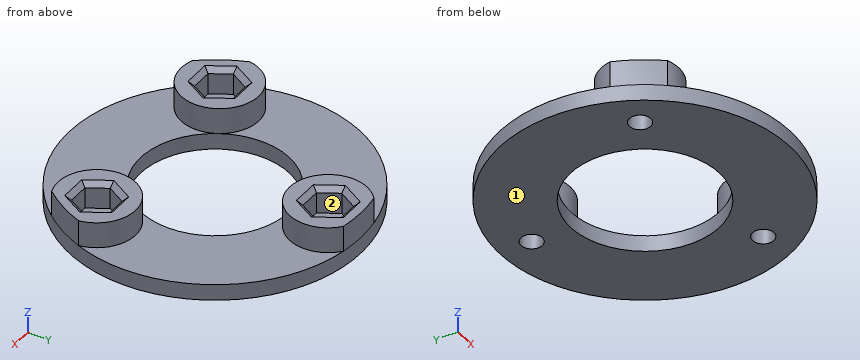
from build123d import *

# Parameters (mm, degrees)
SKETCH1_R           = 22.5
SKETCH1_R_2         = 11.5
SKETCH1_R_3         = 1.65
BOSS_EXTRUDE1_DEPTH = 2.5
BOSS_EXTRUDE2_DEPTH = 4
CHAMFER1_SIZE       = 0.75


with BuildPart() as part:
    # Sketch1 → Boss-Extrude1 (new body)
    with BuildSketch(Plane.XY):
        Circle(SKETCH1_R)
        Circle(SKETCH1_R_2, mode=Mode.SUBTRACT)
        with Locations((0, 17.5)):
            Circle(SKETCH1_R_3, mode=Mode.SUBTRACT)
        with Locations((15.155444566, -8.75)):
            Circle(SKETCH1_R_3, mode=Mode.SUBTRACT)
        with Locations((-15.155444566, -8.75)):
            Circle(SKETCH1_R_3, mode=Mode.SUBTRACT)
    extrude(amount=BOSS_EXTRUDE1_DEPTH)

    # Sketch2 → Boss-Extrude2 (add)
    # profile 1 of 3: a face of its own
    with BuildSketch(Plane.XY.offset(2.5)):
        with BuildLine():
            ThreePointArc((3.747543413, 22.185714286), (0, 22.5), (-3.747543413, 22.185714286))
            ThreePointArc((-3.747543413, 22.185714286), (0, 11.5), (3.747543413, 22.185714286))
        make_face()
        Polygon((1.659882024, 20.375), (3.319764048, 17.5), (1.659882024, 14.625), (-1.659882024, 14.625), (-3.319764048, 17.5), (-1.659882024, 20.375), align=None, mode=Mode.SUBTRACT)
    # profile 2 of 3: a face of its own
    with BuildSketch(Plane.XY.offset(2.5)):
        with BuildLine():
            ThreePointArc((-17.339620466, -14.33832494), (-9.959292144, -5.75), (-21.087163879, -7.847389345))
            ThreePointArc((-21.087163879, -7.847389345), (-19.485571585, -11.25), (-17.339620466, -14.33832494))
        make_face()
        Polygon((-18.475208614, -8.75), (-16.81532659, -5.875), (-13.495562542, -5.875), (-11.835680518, -8.75), (-13.495562542, -11.625), (-16.81532659, -11.625), align=None, mode=Mode.SUBTRACT)
    # profile 3 of 3: a face of its own
    with BuildSketch(Plane.XY.offset(2.5)):
        with BuildLine():
            ThreePointArc((17.339620466, -14.33832494), (19.485571585, -11.25), (21.087163879, -7.847389345))
            ThreePointArc((21.087163879, -7.847389345), (9.959292144, -5.75), (17.339620466, -14.33832494))
        make_face()
        Polygon((16.81532659, -11.625), (13.495562542, -11.625), (11.835680518, -8.75), (13.495562542, -5.875), (16.81532659, -5.875), (18.475208614, -8.75), align=None, mode=Mode.SUBTRACT)
    extrude(amount=BOSS_EXTRUDE2_DEPTH)

    # Chamfer1
    chamfer1_edges = [part.edges().sort_by_distance(p)[0] for p in [
        (2.489823036, 16.0625, 6.5),
        (0, 14.625, 6.5),
        (-2.489823036, 16.0625, 6.5),
        (-2.489823036, 18.9375, 6.5),
        (0, 20.375, 6.5),
        (2.489823036, 18.9375, 6.5),
        (-15.155444566, -5.875, 6.5),
        (-12.66562153, -7.3125, 6.5),
        (-12.66562153, -10.1875, 6.5),
        (-15.155444566, -11.625, 6.5),
        (-17.645267602, -10.1875, 6.5),
        (-17.645267602, -7.3125, 6.5),
        (12.66562153, -10.1875, 6.5),
        (12.66562153, -7.3125, 6.5),
        (15.155444566, -5.875, 6.5),
        (17.645267602, -7.3125, 6.5),
        (17.645267602, -10.1875, 6.5),
        (15.155444566, -11.625, 6.5),
    ]]
    chamfer(chamfer1_edges, length=CHAMFER1_SIZE)


solid = part.part
Work out the finished part from the listing and answer in its coordinate system (mm). Face numbers are marked on the shaded views. A direction names the side the tool comes from. Give positions to 0.01 mm unless a question says otherwise; leave off trailing zeros. Loops run counter-clockwise (first coordinate to the right, second up) from the corner with the lowest first, then second, coordinate; pieces in that order, holes last. Notation, with made-up numbers: M 14.25,-1.5 L 36.25,-1.5 A12 cw 36.25,15.5 Z; hole C -24,11.5 d6. An arc over 180 degrees is marked long. Use CSV: the item, a comma, the result in double quotes.
1) Find section B-B on y = 8. Write down the section's boundary in (x, z), plus the area to 3 significant figures.
Answer:
outline,"M -21.03,0 L -8.26,0 L -8.26,2.5 L -21.03,2.5 Z; M 8.26,0 L 21.03,0 L 21.03,2.5 L 8.26,2.5 Z"
area,"63.8 mm^2"
2) Consider L1, parallel to Y at x = 0, z = 0.7; L2, parallel to Y at x = -15, z = 3 (3 decimals); L3, parallel to Y at x = 0, z = 3.5 (3 decimals). Determine where each line is inside the solid, lowest interval first.
Answer:
L1,"-22.5 to -11.5, 11.5 to 15.85, 19.15 to 22.5"
L2,"-14.748 to -11.625, -5.875 to -2.752"
L3,"11.5 to 14.625, 20.375 to 22.5"
3) Find section A-A on z = 1.75. Write down the section's boundary in (x, y).
Answer:
outline,"C 0,0 d45; hole C -15.16,-8.75 d3.3; hole C 0,0 d23; hole C 0,17.5 d3.3; hole C 15.16,-8.75 d3.3"
4) Find section D-D on y = -1.5. Write down the section's boundary in (x, z), plus the area to 3 significant figures.
Answer:
outline,"M -22.45,0 L -11.4,0 L -11.4,2.5 L -22.45,2.5 Z; M 11.4,0 L 22.45,0 L 22.45,2.5 L 11.4,2.5 Z"
area,"55.2 mm^2"
5) Find section C-C on y = -9.5. Give the number of separate pieces and of enclosed holes in the cut face, plus the area to 3 significant figures.
Answer:
separate pieces,"4"
enclosed holes,"0"
area,"96.9 mm^2"
6) Which of the six approach directions +Z, -Z, +X, -X, +Y, -Y give full straight-line access (tool end or side, diameter ignored) to the marked faces 1 and 2?
Answer:
face 1,"-Z, +X, -X, +Y, -Y"
face 2,"+Z"
7) Given P1, Ø3.5, axis at x = -15, z = 3.5, coming from the -Y side; P2, Ø1.6, axis at x = 15.5, z = 5, coming from the -Y side; P3, Ø11.5, axis at x = -8.5, y = 5.5, coming from the +Z side; P4, Ø2.5, axis at x = -15.16, y = -8.75, coming from the +Z side, each flat-ended and moving along its own axis, determine where each tip first touches the part or whether it passes through.
Answer:
P1,"y = -17.95"
P2,"y = -14.75"
P3,"z = 2.5"
P4,"through"
